from build123d import *

# Parameters (mm, degrees)
SKETCH1_R           = 3.175
BOSS_EXTRUDE1_DEPTH = 6.35
SKETCH2_R           = 3.175
BOSS_EXTRUDE2_DEPTH = 3.81
BOSS_EXTRUDE3_START = -10.16
SKETCH2_2_R         = 3.175
BOSS_EXTRUDE3_DEPTH = 3.81
SKETCH4_R           = 3.175
BOSS_EXTRUDE4_DEPTH = 8.89


with BuildPart() as part:
    # Sketch1 → Boss-Extrude1 (new body)
    with BuildSketch(Plane.XY):
        with BuildLine():
            Line((-5.715, 0), (-5.715, -41.682099171))
            ThreePointArc((-5.715, -41.682099171), (0, -50.8), (5.715, -41.682099171))
            Line((5.715, -41.682099171), (5.715, 0))
            ThreePointArc((5.715, 0), (0, 5.715), (-5.715, 0))
        make_face()
        Circle(SKETCH1_R, mode=Mode.SUBTRACT)
    extrude(amount=BOSS_EXTRUDE1_DEPTH)

    # Sketch2 → Boss-Extrude2 (add)
    with BuildSketch(Plane.XY.offset(6.35)):
        with Locations(Location((0, -47.625, 0), (0, 0, 269.999356937))):
            Circle(SKETCH2_R)
    extrude(amount=BOSS_EXTRUDE2_DEPTH)

    # Sketch2<2> → Boss-Extrude3 (add)
    with BuildSketch(Plane.XY.offset(6.35).offset(BOSS_EXTRUDE3_START)):
        with Locations(Location((0, -47.625, 0), (0, 0, 269.999356937))):
            Circle(SKETCH2_2_R)
    extrude(amount=BOSS_EXTRUDE3_DEPTH)

    # Sketch4 → Boss-Extrude4 (add)
    with BuildSketch(Plane.XY.offset(6.35)):
        with BuildLine():
            Line((-5.715, -8.89), (5.715, -8.89))
            Line((5.715, -8.89), (5.715, 0))
            ThreePointArc((5.715, 0), (0, 5.715), (-5.715, 0))
            Line((-5.715, 0), (-5.715, -8.89))
        make_face()
        Circle(SKETCH4_R, mode=Mode.SUBTRACT)
    extrude(amount=BOSS_EXTRUDE4_DEPTH)


solid = part.part
Design review of the part built by this model. Coordinates are the model's own, in mm. A direction names the side the tool comes from. Round coordinates to 2 decimals unless told otherwise and drop trailing zeros. Write each loop counter-clockwise with the first axis right and the second up, starting at its lowest first coordinate (ties: lowest second). Pieces come first, ordered by that corner, then holes.
Item 1: Draft analysis for pull direction Y (two halves, no side actions). For faces 4 (the flat face through (0, -48, 10.16)), 5 (the cylindrical face through (0.14, -44.453, -1.932)), 6 (the cylindrical face through (0.126, 5.714, 7.513)), 7 (the flat face through (0, -8.89, 11)), state which applies: released by +Y, released by -Y, zero draft, split by the parting line, or undercut.
Item 2: For faces 1 (the flat face through (5.715, -17, 4)), 2 (the flat face through (-5.715, -16, 4)), 3 (the cylindrical face through (0.14, -44.453, 8.228)), list the 3-axis set-ups (+Z, -Z, +X, -X, +Y, -Y) from which the entire face can be reached by the end or side of a thin tool; tool diameter is ignored.
Item 3: Consider section B-B on z = 8.75. Give the boundary of the cut face in (x, y) (3 decimals), and give its area (3 significant figures).
Item 4: Consider section C-C on y = -19.5. Give the boundary of the cut face in (x, z) (3 decimals).
Item 5: Consider section A-A on z = 4. Give the boundary of the cut face in (x, y) (3 decimals).
Item 6: Wall thickness on L1, parallel to Y at x = 0, z = 9.25 (3 decimals); L2, parallel to Y at x = 0, z = 4.5 (3 decimals); L3, parallel to X at y = -21.5, z = 1 (3 decimals): over which ranges is each line inside the solid? List them lowest first.
Item 7: For pin 1 Ø3 at (y, z) = (-3, 2.5) entering from +X (3 decimals); pin 2 Ø5 at (x, z) = (-3, 8) entering from +Y; pin 3 Ø2 at (x, y) = (-0.5, -32) entering from +Z; pin 4 Ø5.5 at (x, y) = (0, 0) entering from -Z, all flat-tipped, find the tip position at first contact; note any pin that passes through.
Item 8: Consider section D-D on x = 3.75. Give the boundary of the cut face in (y, z).
Check values:
1. face 4: zero draft
1. face 5: split by the parting line
1. face 6: released by +Y
1. face 7: undercut
2. face 1: +Z, -Z, +X, +Y
2. face 2: +Z, -Z, -X, +Y
2. face 3: +Z
3. outline: (-5.715, -8.89) - (5.715, -8.89) - (5.715, 0) arc R5.715 ccw to (-5.715, 0) - close; circle Ø6.35 at (0, -47.625); hole circle Ø6.35 at (0, 0)
3. area: 153 mm2
4. outline: (-5.715, 0) - (5.715, 0) - (5.715, 6.35) - (-5.715, 6.35) - close
5. outline: (-5.715, -41.682) arc R6.35 ccw (long way) to (5.715, -41.682) - (5.715, 0) arc R5.715 ccw to (-5.715, 0) - close; hole circle Ø6.35 at (0, 0)
6. L1: y = -50.8 to -44.45, -8.89 to -3.175, 3.175 to 5.715
6. L2: y = -50.8 to -3.175, 3.175 to 5.715
6. L3: x = -5.715 to 5.715
7. pin 1: stops at x = 5.715
7. pin 2: stops at y = 5.69
7. pin 3: stops at z = 6.35
7. pin 4: passes through
8. outline: (-49.57, 0) - (4.31, 0) - (4.31, 15.24) - (-8.89, 15.24) - (-8.89, 6.35) - (-49.57, 6.35) - close
